```python
from build123d import *

# Parameters (mm, degrees)
SKETCH1_R           = 66
BOSS_EXTRUDE1_DEPTH = 1.5
SKETCH2_R           = 63.4
BOSS_EXTRUDE2_DEPTH = 2.5
SKETCH3_R           = 54.6
CUT_EXTRUDE1_DEPTH  = 10
SKETCH4_R           = 1.6
CUT_EXTRUDE2_DEPTH  = 10
SKETCH5_R           = 3
CUT_EXTRUDE3_DEPTH  = 3


with BuildPart() as part:
    # Sketch1 → Boss-Extrude1 (new body)
    with BuildSketch(Plane.XY):
        Circle(SKETCH1_R)
    extrude(amount=BOSS_EXTRUDE1_DEPTH)

    # Sketch2 → Boss-Extrude2 (add)
    with BuildSketch(Plane.XY.offset(1.5)):
        Circle(SKETCH2_R)
    extrude(amount=BOSS_EXTRUDE2_DEPTH)

    # Sketch3 → Cut-Extrude1 (cut)
    with BuildSketch(Plane.XY.offset(4)):
        Circle(SKETCH3_R)
    extrude(amount=-CUT_EXTRUDE1_DEPTH, mode=Mode.SUBTRACT)

    # Sketch4 → Cut-Extrude2 (cut)
    with BuildSketch(Plane.XY.offset(4)):
        with Locations((0, 60.5)):
            Circle(SKETCH4_R)
        with Locations((52.394536929, 30.25)):
            Circle(SKETCH4_R)
        with Locations((52.394536929, -30.25)):
            Circle(SKETCH4_R)
        with Locations((0, -60.5)):
            Circle(SKETCH4_R)
        with Locations((-52.394536929, -30.25)):
            Circle(SKETCH4_R)
        with Locations((-52.394536929, 30.25)):
            Circle(SKETCH4_R)
    extrude(amount=-CUT_EXTRUDE2_DEPTH, mode=Mode.SUBTRACT)

    # Sketch5 → Cut-Extrude3 (cut)
    with BuildSketch(Plane(origin=(0, 0, 0), x_dir=(-1, 0, 0), z_dir=(0, 0, -1))):
        with Locations((-52.394536929, 30.25)):
            Circle(SKETCH5_R)
        with Locations((0, 60.5)):
            Circle(SKETCH5_R)
        with Locations((-52.394536929, -30.25)):
            Circle(SKETCH5_R)
        with Locations((0, -60.5)):
            Circle(SKETCH5_R)
        with Locations((52.394536929, -30.25)):
            Circle(SKETCH5_R)
        with Locations((52.394536929, 30.25)):
            Circle(SKETCH5_R)
    extrude(amount=-CUT_EXTRUDE3_DEPTH, mode=Mode.SUBTRACT)


solid = part.part
```
For this review, take the finished solid that the model builds, in its own axes (mm). A direction names the side the tool comes from. Round coordinates to 2 decimals unless told otherwise and drop trailing zeros. Write each loop counter-clockwise with the first axis right and the second up, starting at its lowest first coordinate (ties: lowest second). Pieces come first, ordered by that corner, then holes. Notation, with made-up numbers: (71, -31.75) -> (79, -31.75) arc R22 ccw to (79, -1.75) -> close; hole circle Ø2 at (56.25, -39). An arc over 180 degrees is marked (long way). One line per question, with ' | ' between items. Start each with the question number.
(1) Add section D-D, the plane y = -60.5. Write out the cut boundary in (x, z).
(2) For line 1 along Y through (x, z) = (0, 0.6); line 2 along Y through (x, z) = (0, 3.7); line 3 along X through (y, z) = (30.25, 1), list the stretches that pass through material, from the lowest coordinate up. Write a range as from..to.
(3) Add section C-C, the plane z = 2.4. Write out the cut boundary in (x, y), plus the area to 3 significant figures.
(4) Add section B-B, the plane x = 12.5. Write out the cut boundary in (y, z), plus the area to 3 significant figures.
(5) Add section A-A, the plane y = 0. Write out the cut boundary in (x, z).
(6) Tool access review of faces 1 (the face through (-50.87, 30.73, 3.51)), 2 (the face through (-25, 59, 1.5)), 3 (the face through (-1, -62, 3)): name each direction out of +Z, -Z, +X, -X, +Y, -Y from which nothing blocks a thin tool from reaching the whole face with its end or side.
(7) Insertion check: P1, Ø1, axis at x = 45.5, z = 1.5, coming from the +Y side; P2, Ø8, axis at x = -52.39, y = 30.25, coming from the +Z side; P3, Ø4, axis at x = -52.39, y = 30.25, coming from the -Z side; P4, Ø1.5, axis at x = 41, z = 3.5, coming from the +Y side. Each pin has a flat end and moves straight along its axis. Give the tip position at first contact, or say it passes through.
Answer list:
1) outline: (-26.38, 0) -> (-3, 0) -> (-3, 3) -> (-1.6, 3) -> (-1.6, 4) -> (-18.96, 4) -> (-18.96, 1.5) -> (-26.38, 1.5) -> close; (1.6, 3) -> (3, 3) -> (3, 0) -> (26.38, 0) -> (26.38, 1.5) -> (18.96, 1.5) -> (18.96, 4) -> (1.6, 4) -> close
2) line 1: -66..-63.5, -57.5..-54.6, 54.6..57.5, 63.5..66 | line 2: -63.4..-62.1, -58.9..-54.6, 54.6..58.9, 62.1..63.4 | line 3: -58.66..-55.39, -49.39..-45.45, 45.45..49.39, 55.39..58.66
3) outline: (-55.29, -31.02) arc R3 cw (long way) to (-54.51, -32.38) arc R63.4 ccw to (-0.79, -63.4) arc R3 cw (long way) to (0.79, -63.4) arc R63.4 ccw to (54.51, -32.38) arc R3 cw (long way) to (55.29, -31.02) arc R63.4 ccw to (55.29, 31.02) arc R3 cw (long way) to (54.51, 32.38) arc R63.4 ccw to (0.79, 63.4) arc R3 cw (long way) to (-0.79, 63.4) arc R63.4 ccw to (-54.51, 32.38) arc R3 cw (long way) to (-55.29, 31.02) arc R63.4 ccw to start; hole circle Ø109.2 at (0, 0) | area: 3,090 mm²
4) outline: (-64.81, 0) -> (-53.15, 0) -> (-53.15, 4) -> (-62.16, 4) -> (-62.16, 1.5) -> (-64.81, 1.5) -> close; (53.15, 0) -> (64.81, 0) -> (64.81, 1.5) -> (62.16, 1.5) -> (62.16, 4) -> (53.15, 4) -> close | area: 80.0 mm²
5) outline: (-66, 0) -> (-54.6, 0) -> (-54.6, 4) -> (-63.4, 4) -> (-63.4, 1.5) -> (-66, 1.5) -> close; (54.6, 0) -> (66, 0) -> (66, 1.5) -> (63.4, 1.5) -> (63.4, 4) -> (54.6, 4) -> close
6) face 1: +Z, -Z | face 2: +Z | face 3: -Z
7) P1: y = 48.28 | P2: z = 4 | P3: z = 3 | P4: y = 48.98
